```python
from build123d import *

# Parameters (mm, degrees)
SKETCH_1_R          = 35
SKETCH_1_R_2        = 1.5
EXTRUDE_1_DEPTH     = 1
SKETCH_2_W          = 6
SKETCH_2_H          = 32
SKETCH_2_R          = 1.5
EXTRUDE_2_DEPTH     = 1
SKETCH_3_R          = 35
CUT_EXTRUDE_1_DEPTH = 1


with BuildPart() as part:
    # Эскиз1 → Бобышка-Вытянуть1 (new body)
    with BuildSketch(Plane(origin=(0, 0, 0), x_dir=(1, 0, 0), z_dir=(0, 1, 0))):
        with Locations(Location((0, 0, 0), (0, 0, 270))):
            Circle(SKETCH_1_R)
        with BuildLine():
            Line((-20.493901532, -16), (20.493901532, -16))
            ThreePointArc((20.493901532, -16), (0, -26), (-20.493901532, -16))
        make_face(mode=Mode.SUBTRACT)
        with BuildLine():
            Line((-18, -10), (-24, -10))
            ThreePointArc((-24, -10), (-26, 0), (-24, 10))
            Line((-24, 10), (-18, 10))
            Line((-18, 10), (24, 10))
            ThreePointArc((24, 10), (26, 0), (24, -10))
            Line((24, -10), (-18, -10))
        make_face(mode=Mode.SUBTRACT)
        with Locations(Location((-18, -13, 0), (0, 0, 270))):
            Circle(SKETCH_1_R_2, mode=Mode.SUBTRACT)
        with Locations(Location((-9, -13, 0), (0, 0, 270))):
            Circle(SKETCH_1_R_2, mode=Mode.SUBTRACT)
        with Locations(Location((0, -13, 0), (0, 0, 270))):
            Circle(SKETCH_1_R_2, mode=Mode.SUBTRACT)
        with Locations(Location((9, -13, 0), (0, 0, 270))):
            Circle(SKETCH_1_R_2, mode=Mode.SUBTRACT)
        with Locations(Location((18, -13, 0), (0, 0, 270))):
            Circle(SKETCH_1_R_2, mode=Mode.SUBTRACT)
        with Locations(Location((-21.566756826, -21.566756826, 0), (0, 0, 270))):
            Circle(SKETCH_1_R_2, mode=Mode.SUBTRACT)
        with Locations(Location((-30.5, 0, 0), (0, 0, 270))):
            Circle(SKETCH_1_R_2, mode=Mode.SUBTRACT)
        with Locations(Location((0, -30.5, 0), (0, 0, 270))):
            Circle(SKETCH_1_R_2, mode=Mode.SUBTRACT)
        with Locations(Location((21.566756826, -21.566756826, 0), (0, 0, 270))):
            Circle(SKETCH_1_R_2, mode=Mode.SUBTRACT)
        with Locations(Location((-21.566756826, 21.566756826, 0), (0, 0, 270))):
            Circle(SKETCH_1_R_2, mode=Mode.SUBTRACT)
        with BuildLine():
            ThreePointArc((-20.493901532, 16), (0, 26), (20.493901532, 16))
            Line((20.493901532, 16), (-20.493901532, 16))
        make_face(mode=Mode.SUBTRACT)
        with Locations(Location((0, 30.5, 0), (0, 0, 270))):
            Circle(SKETCH_1_R_2, mode=Mode.SUBTRACT)
        with Locations(Location((21.566756826, 21.566756826, 0), (0, 0, 270))):
            Circle(SKETCH_1_R_2, mode=Mode.SUBTRACT)
        with Locations(Location((30.5, 0, 0), (0, 0, 270))):
            Circle(SKETCH_1_R_2, mode=Mode.SUBTRACT)
        with Locations(Location((18, 13, 0), (0, 0, 270))):
            Circle(SKETCH_1_R_2, mode=Mode.SUBTRACT)
        with Locations(Location((-18, 13, 0), (0, 0, 270))):
            Circle(SKETCH_1_R_2, mode=Mode.SUBTRACT)
        with Locations(Location((-9, 13, 0), (0, 0, 270))):
            Circle(SKETCH_1_R_2, mode=Mode.SUBTRACT)
        with Locations(Location((0, 13, 0), (0, 0, 270))):
            Circle(SKETCH_1_R_2, mode=Mode.SUBTRACT)
        with Locations(Location((9, 13, 0), (0, 0, 270))):
            Circle(SKETCH_1_R_2, mode=Mode.SUBTRACT)
    extrude(amount=EXTRUDE_1_DEPTH)

    # Эскиз2 → Бобышка-Вытянуть2 (add)
    with BuildSketch(Plane(origin=(0, 1, 0), x_dir=(1, 0, 0), z_dir=(0, 1, 0))):
        with Locations((-9, 0)):
            Rectangle(SKETCH_2_W, SKETCH_2_H)
        with Locations(Location((-9, -7.5, 0), (0, 0, 270))):
            Circle(SKETCH_2_R, mode=Mode.SUBTRACT)
        with Locations(Location((-9, 7.5, 0), (0, 0, 270))):
            Circle(SKETCH_2_R, mode=Mode.SUBTRACT)
        with Locations(Location((-9, -13, 0), (0, 0, 270))):
            Circle(SKETCH_2_R, mode=Mode.SUBTRACT)
        with Locations(Location((-9, 13, 0), (0, 0, 270))):
            Circle(SKETCH_2_R, mode=Mode.SUBTRACT)
    extrude(amount=EXTRUDE_2_DEPTH)

    # Эскиз3 → Вырез-Вытянуть1 (cut)
    with BuildSketch(Plane.XZ):
        Circle(SKETCH_3_R)
    extrude(amount=-CUT_EXTRUDE_1_DEPTH, mode=Mode.SUBTRACT)


solid = part.part
```
Model file for the job. Use its own axes, mm. Coordinates: 2 decimals unless noted, no trailing zeros. Order: outer loops, then holes, each group sorted by start corner. A loop starts at its lowest first (then second) coordinate and runs counter-clockwise, first axis right, second up. Notation, with made-up numbers: (-17, 76.25) -> (-3, 76.25) arc R29 cw to (-3, 113.25) -> close; hole circle Ø10 at (53.25, 2.25). An arc over 180 degrees is marked (long way). Return JSON: item names as keys, results as strings.
Item 1: Mould opens along Z. For faces 1 (the face through (-6, 1.5, 0.2)), 2 (the face through (-9.9, 1.5, 11.8)), 3 (the face through (-9, 1.5, 16)), 4 (the face through (-9.9, 1.5, -8.7)) say: pulls with the +Z half, pulls with the -Z half, needs draft (parallel to the pull), parting line crosses it, or undercut.
Model answer:
{"face 1": "needs draft", "face 2": "undercut", "face 3": "pulls with the +Z half", "face 4": "undercut"}
Item 2: Slice it at C-C (y = 1.45). Write the cut outline in (x, z), then the cut area to 3 significant figures.
Model answer:
{"outline": "(-12, -16) -> (-6, -16) -> (-6, 16) -> (-12, 16) -> close; hole circle Ø3 at (-9, -13); hole circle Ø3 at (-9, -7.5); hole circle Ø3 at (-9, 7.5); hole circle Ø3 at (-9, 13)", "area": "164 mm²"}
Item 3: Slice it at D-D (x = -9.9). Write the cut outline in (y, z), then the cut area to 3 significant figures.
Model answer:
{"outline": "(1, -16) -> (2, -16) -> (2, -14.2) -> (1, -14.2) -> close; (1, -11.8) -> (2, -11.8) -> (2, -8.7) -> (1, -8.7) -> close; (1, -6.3) -> (2, -6.3) -> (2, 6.3) -> (1, 6.3) -> close; (1, 8.7) -> (2, 8.7) -> (2, 11.8) -> (1, 11.8) -> close; (1, 14.2) -> (2, 14.2) -> (2, 16) -> (1, 16) -> close", "area": "22.4 mm²"}
Item 4: Slice it at A-A (x = -7.8). Write the cut outline in (y, z), then the cut area to 3 significant figures.
Model answer:
{"outline": "(1, -16) -> (2, -16) -> (2, -13.9) -> (1, -13.9) -> close; (1, -12.1) -> (2, -12.1) -> (2, -8.4) -> (1, -8.4) -> close; (1, -6.6) -> (2, -6.6) -> (2, 6.6) -> (1, 6.6) -> close; (1, 8.4) -> (2, 8.4) -> (2, 12.1) -> (1, 12.1) -> close; (1, 13.9) -> (2, 13.9) -> (2, 16) -> (1, 16) -> close", "area": "24.8 mm²"}
Item 5: Slice it at B-B (z = -7.5). Write the cut outline in (x, y).
Model answer:
{"outline": "(-12, 1) -> (-10.5, 1) -> (-10.5, 2) -> (-12, 2) -> close; (-7.5, 1) -> (-6, 1) -> (-6, 2) -> (-7.5, 2) -> close"}
Item 6: Pin check, flat tip, straight feed: P1, Ø1.8, axis at x = -9, z = -13, coming from the -Y side. Stop position of the tip, or through.
Model answer:
{"P1": "passes through"}
Item 7: Wall check: line 1 along Z through (x, y) = (-9.65, 1.55); line 2 along Z through (x, y) = (-9.35, 1.15); line 3 along X through (y, z) = (1.25, 7.5). Give the ranges that are in metal, low to high. Write a range as from..to.
Model answer:
{"line 1": "z = -16..-14.35, -11.65..-8.85, -6.15..6.15, 8.85..11.65, 14.35..16", "line 2": "z = -16..-14.46, -11.54..-8.96, -6.04..6.04, 8.96..11.54, 14.46..16", "line 3": "x = -12..-10.5, -7.5..-6"}
